Design review of the part built by this model. Coordinates are the model's own, in mm. A direction names the side the tool comes from. Coordinates: 2 decimals unless noted, no trailing zeros. Loops run counter-clockwise (first coordinate to the right, second up) from the corner with the lowest first, then second, coordinate; pieces in that order, holes last. Notation, with made-up numbers: (8, -23.75) - (28, -23.75) arc R15 cw to (28, -14.75) - close; hole circle Ø6 at (13, 88). An arc over 180 degrees is marked (long way). Answer in a Markdown table with one row per item. Add a question column.
(1) To check wall thickness, follow L1, parallel to Y at x = -6, z = 13; L2, parallel to X at y = 15, z = 7.25; L3, parallel to Y at x = -9, z = 10. State the ranges of each line that lie inside material, in increasing order. Write a range as [from, to].
(2) We need section C-C, the plane z = 3.5. Write out the cut boundary in (x, y), plus the area to 3 significant figures.
(3) We need section D-D, the plane z = 22.5. Write out the cut boundary in (x, y).
(4) The part is to be moulded in two halves that separate along X. For faces 5 (the face through (-5.483, 17.133, 12.522)), 6 (the face through (14.9, -17.41, 1.84)), 7 (the face through (-5, 0, 12)), say which applies: released by +X, released by -X, zero draft, split by the parting line, or undercut.
(5) For faces 1 (the face through (1.83, -27.66, 1.84)), 2 (the face through (-4, -12, 2.54)), 3 (the face through (-7.6, -8.8, 1.3)), 4 (the face through (-23.043, -17.405, 1.841)), list the 3-axis set-ups (+Z, -Z, +X, -X, +Y, -Y) from which the entire face can be reached by the end or side of a thin tool; tool diameter is ignored.
(6) Clearance check with flat-ended pins moving along their axes: pin 1 (4.5 mm diameter, centred on x = -5.98, y = 13.36, fed in from -Z); pin 2 (6 mm diameter, centred on x = -10, z = 10.5, fed in from -Y); pin 3 (15.5 mm diameter, centred on x = -3.5, y = -14.5, fed in from +Z); pin 4 (4 mm diameter, centred on x = -5.5, y = 2, fed in from -Z). State where each tip first meets the part, or that it passes through.
(7) We need section A-A, the plane y = 8. Write out the cut boundary in (x, z), plus the area to 3 significant figures.
(8) We need section B-B, the plane x = 7. Write out the cut boundary in (y, z), plus the area to 3 significant figures.
from build123d import *

# Parameters (mm, degrees)
F0_W          = 41.1070454866
F0_H          = 27.6698879898
F1_DEPTH      = 25.4
F2_W          = 41.600080207
F2_H          = 35.3044494987
F3_DEPTH      = 2.54
F5_DEPTH      = 25.4
F7_D          = 7.62
F7_DEPTH      = 508
F7_TIP        = 2.2892789585
F9_D          = 2.54
F9_DEPTH      = 508
F9_TIP        = 0.7630929862
F11_D         = 5.08
F11_DEPTH     = 508
F11_TIP       = 1.5261859723
F12_SIZE      = 5.08
F13_T1_DEPTH  = 46.3029721267
F13_T3_DEPTH  = 38.7218051595
F13_T5_DEPTH  = 33.8444602975
F13_T7_DEPTH  = 23.3607587036
F13_T9_DEPTH  = 0.3279052623
F13_T12_ANGLE = 90
F13_T14_ANGLE = 90


# Not quite as in the source:
# - a fillet or chamfer that OpenCascade refuses, or shapes differently, is made with other operations: its cross-section is extruded or revolved along the edge and cut away or added


with BuildPart() as f1:
    # F0 (on Top) → F1 (new body)
    with BuildSketch(Plane.XY):
        with Locations((-4.3705804273, 13.8349439949)):
            Rectangle(F0_W, F0_H)
    extrude(amount=F1_DEPTH)

    # F2 (on Top) → F3 (join)
    with BuildSketch(Plane.XY):
        with Locations((-4.0700184181, -17.6522247493)):
            Rectangle(F2_W, F2_H)
    extrude(amount=F3_DEPTH)

    # F4 (on face) → F5 (cut)
    with BuildSketch(Plane.XY.offset(2.54)):
        with BuildLine():
            Line((-13.0226434802, -22.9422134231), (-13.0226434802, -45.534973538))
            Line((-13.0226434802, -45.534973538), (0.005261782, -45.534973538))
            Line((0.005261782, -45.534973538), (0.005261782, -22.9422134231))
            ThreePointArc((0.005261782, -22.9422134231), (-1.8546101574, -18.4520853626), (-6.344738218, -16.5922134231))
            Line((-6.344738218, -16.5922134231), (-6.6726434802, -16.5922134231))
            ThreePointArc((-6.6726434802, -16.5922134231), (-11.1627715408, -18.4520853626), (-13.0226434802, -22.9422134231))
        make_face()
    extrude(amount=-F5_DEPTH, mode=Mode.SUBTRACT)

    # F7
    with Locations(Plane.XY.offset(25.4)):
        with Locations((-5.9787402861, 13.3550977334)):
            Hole(F7_D / 2, depth=F7_DEPTH)
            with Locations((0, 0, -(F7_DEPTH + F7_TIP / 2))):  # 118° drill point
                Cone(0, F7_D / 2, F7_TIP, mode=Mode.SUBTRACT)

    # F9
    with Locations(Plane.XY.offset(2.54)):
        with Locations((-6.6726434802, -14.2427943647)):
            Hole(F9_D / 2, depth=F9_DEPTH)
            with Locations((0, 0, -(F9_DEPTH + F9_TIP / 2))):  # 118° drill point
                Cone(0, F9_D / 2, F9_TIP, mode=Mode.SUBTRACT)

    # F11
    with Locations(Plane.XY.offset(2.54)):
        with Locations((-6.4694355242, -6.5277060494)):
            Hole(F11_D / 2, depth=F11_DEPTH)
            with Locations((0, 0, -(F11_DEPTH + F11_TIP / 2))):  # 118° drill point
                Cone(0, F11_D / 2, F11_TIP, mode=Mode.SUBTRACT)

    # F12
    f12_edges = [f1.edges().sort_by_distance(p)[0] for p in [
        (-4.37058, 0, 25.4),
        (16.182942, 13.834944, 25.4),
        (-4.37058, 27.669888, 25.4),
        (-24.924103, 13.834944, 25.4),
    ]]
    chamfer(f12_edges, length=F12_SIZE)

    # F13: fillet of radius 5.08 on 5 edges, made by hand

    # F13_s2 → F13_t1 (cut)
    with BuildSketch(Plane.XZ):
        with BuildLine():
            ThreePointArc((16.7300216854, 0), (14.8706126341, 1.8594090512), (12.3306126341, 2.54))
            Line((12.3306126341, 2.54), (16.7300216854, 2.54))
            Line((16.7300216854, 2.54), (16.7300216854, 0))
        make_face()
        with BuildLine():
            ThreePointArc((-24.8700585216, 0), (-23.0106494704, 1.8594090512), (-20.4706494704, 2.54))
            Line((-20.4706494704, 2.54), (-24.8700585216, 2.54))
            Line((-24.8700585216, 2.54), (-24.8700585216, 0))
        make_face()
    extrude(amount=F13_T1_DEPTH, mode=Mode.SUBTRACT)

    # F13_s4 → F13_t3 (cut)
    with BuildSketch(Plane.YZ.offset(-10.993260846)):
        with BuildLine():
            ThreePointArc((-35.3044494987, 0), (-33.4450404474, 1.8594090512), (-30.9050404474, 2.54))
            Line((-30.9050404474, 2.54), (-35.3044494987, 2.54))
            Line((-35.3044494987, 2.54), (-35.3044494987, 0))
        make_face()
    extrude(amount=F13_T3_DEPTH, mode=Mode.SUBTRACT)

    # F13_s6 → F13_t5 (cut)
    with BuildSketch(Plane.YZ.offset(-35.8685811497)):
        with BuildLine():
            ThreePointArc((-35.3044494987, 0), (-33.4450404474, 1.8594090512), (-30.9050404474, 2.54))
            Line((-30.9050404474, 2.54), (-35.3044494987, 2.54))
            Line((-35.3044494987, 2.54), (-35.3044494987, 0))
        make_face()
    extrude(amount=F13_T5_DEPTH, mode=Mode.SUBTRACT)

    # F13_s8 → F13_t7 (cut)
    with BuildSketch(Plane.XZ.offset(22.9422134231)):
        with BuildLine():
            ThreePointArc((0.005261782, 0), (1.8646708333, 1.8594090512), (4.4046708333, 2.54))
            Line((4.4046708333, 2.54), (0.005261782, 2.54))
            Line((0.005261782, 2.54), (0.005261782, 0))
        make_face()
        with BuildLine():
            ThreePointArc((-13.0226434802, 0), (-14.8820525315, 1.8594090512), (-17.4220525315, 2.54))
            Line((-17.4220525315, 2.54), (-13.0226434802, 2.54))
            Line((-13.0226434802, 2.54), (-13.0226434802, 0))
        make_face()
    extrude(amount=F13_T7_DEPTH, mode=Mode.SUBTRACT)

    # F13_s10 → F13_t9 (cut)
    with BuildSketch(Plane.YZ.offset(-6.6726434802)):
        with BuildLine():
            ThreePointArc((-16.5922134231, 0), (-14.7328043719, 1.8594090512), (-12.1928043719, 2.54))
            Line((-12.1928043719, 2.54), (-16.5922134231, 2.54))
            Line((-16.5922134231, 2.54), (-16.5922134231, 0))
        make_face()
    extrude(amount=F13_T9_DEPTH, mode=Mode.SUBTRACT)

    # F13_s11 → F13_t12 (revolve, cut)
    with BuildSketch(Plane.XZ.offset(22.9422134231)):
        with BuildLine():
            ThreePointArc((0.005261782, 0), (1.8646708333, 1.8594090512), (4.4046708333, 2.54))
            Line((4.4046708333, 2.54), (0.005261782, 2.54))
            Line((0.005261782, 2.54), (0.005261782, 0))
        make_face()
    revolve(axis=Axis((-6.344738218, -22.9422134231, 2.54), (0, 0, 1)), revolution_arc=F13_T12_ANGLE, mode=Mode.SUBTRACT)

    # F13_s13 → F13_t14 (revolve, cut)
    with BuildSketch(Plane.YZ.offset(-6.6726434802)):
        with BuildLine():
            ThreePointArc((-16.5922134231, 0), (-14.7328043719, 1.8594090512), (-12.1928043719, 2.54))
            Line((-12.1928043719, 2.54), (-16.5922134231, 2.54))
            Line((-16.5922134231, 2.54), (-16.5922134231, 0))
        make_face()
    revolve(axis=Axis((-6.6726434802, -22.9422134231, 2.54), (0, 0, 1)), revolution_arc=F13_T14_ANGLE, mode=Mode.SUBTRACT)


solid = f1.part
Responses:
| question | item | result |
|---|---|---|
| 1 | L1 | y = [0, 9.55], [17.17, 27.67] |
| 1 | L2 | x = [-24.92, -9.42], [-2.54, 16.18] |
| 1 | L3 | y = [0, 11.03], [15.68, 27.67] |
| 2 | outline | (-24.92, 0) - (16.18, 0) - (16.18, 27.67) - (-24.92, 27.67) - close; hole circle Ø7.62 at (-5.98, 13.36) |
| 2 | area | 1,090 mm2 |
| 3 | outline | (-22.74, 2.18) - (14, 2.18) - (14, 25.49) - (-22.74, 25.49) - close; hole circle Ø7.62 at (-5.98, 13.36) |
| 4 | face 5 | undercut |
| 4 | face 6 | released by +X |
| 4 | face 7 | zero draft |
| 5 | face 1 | +Z, -Y |
| 5 | face 2 | +Z, +X, -X, -Y |
| 5 | face 3 | +Z, -Z |
| 5 | face 4 | +Z, -X, -Y |
| 6 | pin 1 | passes through |
| 6 | pin 2 | stops at y = 0 |
| 6 | pin 3 | stops at z = 2.54 |
| 6 | pin 4 | stops at z = 0 |
| 7 | outline | (-24.92, 0) - (16.18, 0) - (16.18, 20.32) - (11.1, 25.4) - (-19.84, 25.4) - (-24.92, 20.32) - close |
| 7 | area | 1,020 mm2 |
| 8 | outline | (-35.3, 0) - (27.67, 0) - (27.67, 20.32) - (22.59, 25.4) - (5.08, 25.4) - (0, 20.32) - (0, 2.54) - (-30.91, 2.54) arc R5.08 ccw to start |
| 8 | area | 763 mm2 |
